Could you check a few things on this model? Use its own coordinates, in mm. A direction names the side the tool comes from. Coordinates: 2 decimals unless noted, no trailing zeros. Loops run counter-clockwise (first coordinate to the right, second up) from the corner with the lowest first, then second, coordinate; pieces in that order, holes last. Notation, with made-up numbers: M 49.5,25 L 84.5,25 A25 ccw 84.5,62 Z; hole C 36,45.25 d9. An arc over 180 degrees is marked long. Write each question's results on one line, items separated by ' | '.
```python
from build123d import *

# Parameters (mm, degrees)
SKETCH1_R           = 1.5
BOSS_EXTRUDE1_DEPTH = 3
BOSS_EXTRUDE2_DEPTH = 5
FILLET1_R           = 2


with BuildPart() as part:
    # Sketch1 → Boss-Extrude1 (new body)
    with BuildSketch(Plane(origin=(0, 0, 0), x_dir=(1, 0, 0), z_dir=(0, 1, 0))):
        with BuildLine():
            Line((0, 0), (0, 20))
            ThreePointArc((0, 20), (0.817293204, 25.108176699), (2.5, 30))
            ThreePointArc((2.5, 30), (6.776610811, 25.394958109), (10, 20))
            Line((10, 20), (10, 0))
            Line((10, 0), (12, 0))
            ThreePointArc((12, 0), (14.121320344, -0.878679656), (15, -3))
            Line((15, -3), (15, -17))
            ThreePointArc((15, -17), (14.121320344, -19.121320344), (12, -20))
            Line((12, -20), (-2, -20))
            ThreePointArc((-2, -20), (-4.121320344, -19.121320344), (-5, -17))
            Line((-5, -17), (-5, -3))
            ThreePointArc((-5, -3), (-4.121320344, -0.878679656), (-2, 0))
            Line((-2, 0), (0, 0))
        make_face()
        with Locations((5, 12)):
            Circle(SKETCH1_R, mode=Mode.SUBTRACT)
    extrude(amount=BOSS_EXTRUDE1_DEPTH)

    # Sketch2 → Boss-Extrude2 (add, symmetric)
    with BuildSketch(Plane(origin=(0, 1.5, 0), x_dir=(1, 0, 0), z_dir=(0, 1, 0))):
        with BuildLine():
            Line((0, 0), (-2, 0))
            ThreePointArc((-2, 0), (-4.121320344, -0.878679656), (-5, -3))
            Line((-5, -3), (-5, -17))
            ThreePointArc((-5, -17), (-4.121320344, -19.121320344), (-2, -20))
            Line((-2, -20), (12, -20))
            ThreePointArc((12, -20), (14.121320344, -19.121320344), (15, -17))
            Line((15, -17), (15, -3))
            ThreePointArc((15, -3), (14.121320344, -0.878679656), (12, 0))
            Line((12, 0), (10, 0))
            Line((10, 0), (0, 0))
        make_face()
    extrude(amount=BOSS_EXTRUDE2_DEPTH, both=True)

    # Fillet1
    fillet1_edges = [part.edges().sort_by_distance(p)[0] for p in [
        (-4.121320344, -3.5, 0.878679656),
        (-5, -3.5, 10),
        (-4.121320344, -3.5, 19.121320344),
        (5, -3.5, 20),
        (14.121320344, -3.5, 19.121320344),
        (15, -3.5, 10),
        (14.121320344, -3.5, 0.878679656),
        (5, -3.5, 0),
        (5, 6.5, 0),
        (-4.121320344, 6.5, 0.878679656),
        (-5, 6.5, 10),
        (-4.121320344, 6.5, 19.121320344),
        (5, 6.5, 20),
        (14.121320344, 6.5, 19.121320344),
        (15, 6.5, 10),
        (14.121320344, 6.5, 0.878679656),
    ]]
    fillet(fillet1_edges, radius=FILLET1_R)


solid = part.part
```
(1) Imagine slicing it at C-C, the plane x = 5. List the corners of the cut face in (y, z) for me.
Reported:
outline: M -3.5,2 A2 ccw -1.5,0 L 0,0 L 0,-10.5 L 3,-10.5 L 3,0 L 4.5,0 A2 ccw 6.5,2 L 6.5,18 A2 ccw 4.5,20 L -1.5,20 A2 ccw -3.5,18 Z; M 0,-27.55 L 3,-27.55 L 3,-13.5 L 0,-13.5 Z
(2) If we mould it in two halves opening along X, with no side actions, what happens to faces 5 (the cylindrical face through (-4.1, 1.54, 0.86)), 6 (the cylindrical face through (6.386, 1.479, -11.425)), 7 (the flat face through (15, 2, 10))? For each: released by +X, released by -X, zero draft, split by the parting line, or undercut.
Reported:
face 5: released by -X | face 6: undercut | face 7: released by +X
(3) Imagine slicing it at D-D, the plane z = 16.5. List the corners of the cut face in (x, y) for me, and give its area (3 significant figures).
Reported:
outline: M -5,-1.5 A2 ccw -3,-3.5 L 13,-3.5 A2 ccw 15,-1.5 L 15,4.5 A2 ccw 13,6.5 L -3,6.5 A2 ccw -5,4.5 Z | area: 197 mm2
(4) Imagine slicing it at A-A, the plane y = 1.25. List the corners of the cut face in (x, z) for me.
Reported:
outline: M -5,3 A3 ccw -2,0 L 0,0 L 0,-20 A30 ccw 2.5,-30 A30 ccw 10,-20 L 10,0 L 12,0 A3 ccw 15,3 L 15,17 A3 ccw 12,20 L -2,20 A3 ccw -5,17 Z; hole C 5,-12 d3
(5) Which directions (+Z, -Z, +X, -X, +Y, -Y) give clear straight access to the entire face, cutting with the end or side of a thin tool? Please do faces 1 (the flat face through (10, 1, -10)), 2 (the flat face through (0, 1, -10)), 3 (the flat face through (5, 3, -15)), 4 (the flat face through (5, 0, -15)).
Reported:
face 1: -Z, +X, +Y, -Y | face 2: -Z, -X, +Y, -Y | face 3: -Z, +X, -X, +Y | face 4: -Z, +X, -X, -Y
(6) Imagine slicing it at B-B, the plane z = -12. List the corners of the cut face in (x, y) for me.
Reported:
outline: M 0,0 L 3.5,0 L 3.5,3 L 0,3 Z; M 6.5,0 L 10,0 L 10,3 L 6.5,3 Z
(7) Please list where these lines run through material, in increasing order: probe 1 along X at (y, z) = (1.9, -12); probe 2 along Y at (x, z) = (5.5, -15); probe 3 along Z at (x, y) = (5, 1.55). Write a range as from..to.
Reported:
probe 1: x = 0..3.5, 6.5..10 | probe 2: y = 0..3 | probe 3: z = -27.55..-13.5, -10.5..20
(8) Will these pins go through, and if not, where does the flat tip stop? P1, Ø3.5, axis at y = 1.5, z = -6, coming from the -X side; P2, Ø5, axis at x = 5, z = -12.5, coming from the +Y side; P3, Ø5, axis at x = 3, z = -18, coming from the -Y side.
Reported:
P1: stops at x = 0 | P2: stops at y = 3 | P3: stops at y = 0
